Here's how the part is built. I have some questions about the finished solid (model axes, mm). A direction names the side the tool comes from. Coordinates: 2 decimals unless noted, no trailing zeros. Loops run counter-clockwise (first coordinate to the right, second up) from the corner with the lowest first, then second, coordinate; pieces in that order, holes last. Notation, with made-up numbers: (27, -38.75) - (40, -38.75) arc R27 cw to (40, -21.75) - close; hole circle Ø8 at (56.25, 87). An arc over 180 degrees is marked (long way). Use a Markdown table: item, result.
```python
from build123d import *

# Parameters (mm, degrees)
F0_R     = 9.525
F1_DEPTH = 25.4
F3_DEPTH = 25.401
F4_DEPTH = 25.4


with BuildPart() as f1:
    # F0 (on Front) → F1 (new body)
    with BuildSketch(Plane.XZ):
        Circle(F0_R)
    extrude(amount=F1_DEPTH)

    # F2 (on face) → F3 (cut, through all)
    with BuildSketch(Plane.XZ.offset(25.4)):
        with BuildLine():
            ThreePointArc((4.7625, 0), (3.367596, 3.367596), (0, 4.7625))
            ThreePointArc((0, 4.7625), (-3.367596, 3.367596), (-4.7625, 0))
            ThreePointArc((-4.7625, 0), (-3.367596, -3.367596), (0, -4.7625))
            ThreePointArc((0, -4.7625), (3.367596, -3.367596), (4.7625, 0))
        make_face()
    extrude(amount=-F3_DEPTH, mode=Mode.SUBTRACT)

    # F2 (on face) → F4 (cut)
    with BuildSketch(Plane.XZ.offset(25.4)):
        with BuildLine():
            Line((4.7625, 0), (4.7625, 4.7625))
            Line((4.7625, 4.7625), (0, 4.7625))
            ThreePointArc((0, 4.7625), (3.367596, 3.367596), (4.7625, 0))
        make_face()
        with BuildLine():
            ThreePointArc((-4.7625, 0), (-3.367596, 3.367596), (0, 4.7625))
            Line((0, 4.7625), (-4.7625, 4.7625))
            Line((-4.7625, 4.7625), (-4.7625, 0))
        make_face()
        with BuildLine():
            Line((4.7625, -4.7625), (4.7625, 0))
            ThreePointArc((4.7625, 0), (3.367596, -3.367596), (0, -4.7625))
            Line((0, -4.7625), (4.7625, -4.7625))
        make_face()
        with BuildLine():
            ThreePointArc((0, -4.7625), (-3.367596, -3.367596), (-4.7625, 0))
            Line((-4.7625, 0), (-4.7625, -4.7625))
            Line((-4.7625, -4.7625), (0, -4.7625))
        make_face()
    extrude(amount=-F4_DEPTH, mode=Mode.SUBTRACT)


solid = f1.part
```
Q1. Will these pins go through, and if not, where does the flat tip stop? P1, Ø1, axis at y = -4.5, z = 5.5, coming from the +X side; P2, Ø1, axis at y = -5.5, z = 1, coming from the +X side; P3, Ø5, axis at x = -6, y = -8, coming from the +Z side.
Check values:
| item | result |
|---|---|
| P1 | x = 8.11 |
| P2 | x = 9.51 |
| P3 | z = 8.86 |
Q2. Which directions (+Z, -Z, +X, -X, +Y, -Y) give clear straight access to the entire face, cutting with the end or side of a thin tool? Please do faces 4 (the face through (0, 0, -6)), 5 (the face through (4.762, -13, 0)).
Check values:
| item | result |
|---|---|
| face 4 | +Z, -Z, +X, -X, +Y |
| face 5 | +Y, -Y |
Q3. Please list where these lines run through material, in increasing order: L1, parallel to Z at x = 0, y = -13 (1 decimal); L2, parallel to X at y = -4, z = 2; L3, parallel to X at y = -22.5, z = -1.25. Write a range as from..to.
Check values:
| item | result |
|---|---|
| L1 | -9.5..-4.8, 4.8..9.5 |
| L2 | -9.31..-4.76, 4.76..9.31 |
| L3 | -9.44..-4.76, 4.76..9.44 |
Q4. I want a section at D-D, the plane x = -8. Write out the boundary of the cut face in (y, z).
Check values:
| item | result |
|---|---|
| outline | (-25.4, -5.17) - (0, -5.17) - (0, 5.17) - (-25.4, 5.17) - close |
Q5. If we mould it in two halves opening along Z, with no side actions, what happens to faces 1 (the face through (-7.559, -12.522, -5.796)), 2 (the face through (0, -25.4, -6)), 3 (the face through (0, -13, -4.762))? For each: pulls with the +Z half, pulls with the -Z half, needs draft (parallel to the pull), parting line crosses it, or undercut.
Check values:
| item | result |
|---|---|
| face 1 | parting line crosses it |
| face 2 | needs draft |
| face 3 | undercut |
Q6. I want a section at A-A, the plane x = 0. Write out the boundary of the cut face in (y, z) (1 decimal), then the cut area to 3 significant figures.
Check values:
| item | result |
|---|---|
| outline | (-25.4, -9.5) - (0, -9.5) - (0, -4.8) - (-25.4, -4.8) - close; (-25.4, 4.8) - (0, 4.8) - (0, 9.5) - (-25.4, 9.5) - close |
| area | 242 mm^2 |
Q7. I want a section at B-B, the plane z = 0. Write out the boundary of the cut face in (x, y) (1 decimal), then the cut area to 3 significant figures.
Check values:
| item | result |
|---|---|
| outline | (-9.5, -25.4) - (-4.8, -25.4) - (-4.8, 0) - (-9.5, 0) - close; (4.8, -25.4) - (9.5, -25.4) - (9.5, 0) - (4.8, 0) - close |
| area | 242 mm^2 |
